```python
from build123d import *

# Parameters (mm, degrees)
SALIENTE_EXTRUIR1_DEPTH = 32
CORTAR_EXTRUIR1_REACH   = 113.66
CROQUIS2_W              = 9.5
CROQUIS2_H              = 13
CORTAR_EXTRUIR2_REACH   = 196.034
REDONDEO2_R             = 16


with BuildPart() as part:
    # Croquis1 → Saliente-Extruir1 (new, symmetric)
    with BuildSketch(Plane.XY):
        with BuildLine():
            Line((-100, 27), (-100, 17))
            Line((-100, 17), (-40, 17))
            Line((-40, 17), (-40, 35))
            ThreePointArc((-40, 35), (-20, 55), (0, 35))
            Line((0, 35), (0, 0))
            Line((0, 0), (80, 0))
            Line((80, 0), (80, 56))
            Line((80, 56), (70, 56))
            Line((70, 56), (70, 10))
            Line((70, 10), (10, 10))
            Line((10, 10), (10, 35))
            ThreePointArc((10, 35), (-20, 65), (-50, 35))
            Line((-50, 35), (-50, 27))
            Line((-50, 27), (-100, 27))
        make_face()
    extrude(amount=SALIENTE_EXTRUIR1_DEPTH, both=True)

    # Croquis2 → Cortar-Extruir1 (cut, up to next)
    with BuildSketch(Plane(origin=(0, 27, 0), x_dir=(1, 0, 0), z_dir=(0, 1, 0)), mode=Mode.PRIVATE) as cortar_extruir1_sk1:
        Polygon((-100, 13.524791386), (-68, 32), (-100, 32), align=None)
    cortar_extruir1_tool1 = extrude(cortar_extruir1_sk1.sketch, amount=-CORTAR_EXTRUIR1_REACH, mode=Mode.PRIVATE) & part.part
    # Croquis2 → Cortar-Extruir1 (cut, up to next)
    with BuildSketch(Plane(origin=(0, 27, 0), x_dir=(1, 0, 0), z_dir=(0, 1, 0)), mode=Mode.PRIVATE) as cortar_extruir1_sk2:
        with Locations((-95.25, 0)):
            Rectangle(CROQUIS2_W, CROQUIS2_H)
    cortar_extruir1_tool2 = extrude(cortar_extruir1_sk2.sketch, amount=-CORTAR_EXTRUIR1_REACH, mode=Mode.PRIVATE) & part.part
    # Croquis2 → Cortar-Extruir1 (cut, up to next)
    with BuildSketch(Plane(origin=(0, 27, 0), x_dir=(1, 0, 0), z_dir=(0, 1, 0)), mode=Mode.PRIVATE) as cortar_extruir1_sk3:
        Polygon((-100, -13.524791386), (-100, -32), (-68, -32), align=None)
    cortar_extruir1_tool3 = extrude(cortar_extruir1_sk3.sketch, amount=-CORTAR_EXTRUIR1_REACH, mode=Mode.PRIVATE) & part.part
    add(cortar_extruir1_tool1.solids().sort_by_distance((-89.333333, 27, -25.841597))[0], mode=Mode.SUBTRACT)
    add(cortar_extruir1_tool2.solids().sort_by_distance((-95.25, 27, 0))[0], mode=Mode.SUBTRACT)
    add(cortar_extruir1_tool3.solids().sort_by_distance((-89.333333, 27, 25.841597))[0], mode=Mode.SUBTRACT)

    # Croquis4 → Cortar-Extruir2 (cut, up to next)
    with BuildSketch(Plane(origin=(80, 0, 0), x_dir=(0, 0, -1), z_dir=(1, 0, 0)), mode=Mode.PRIVATE) as cortar_extruir2_sk1:
        with BuildLine():
            Line((-16, 48.75), (16, 48.75))
            ThreePointArc((16, 48.75), (24.75, 40), (16, 31.25))
            Line((16, 31.25), (-16, 31.25))
            ThreePointArc((-16, 31.25), (-24.75, 40), (-16, 48.75))
        make_face()
    cortar_extruir2_tool1 = extrude(cortar_extruir2_sk1.sketch, amount=-CORTAR_EXTRUIR2_REACH, mode=Mode.PRIVATE) & part.part
    add(cortar_extruir2_tool1.solids().sort_by_distance((80, 40, 0))[0], mode=Mode.SUBTRACT)

    # Redondeo2
    redondeo2_edges = [part.edges().sort_by_distance(p)[0] for p in [
        (75, 56, -32),
        (75, 56, 32),
    ]]
    fillet(redondeo2_edges, radius=REDONDEO2_R)


solid = part.part
```
Input: part model. Units: mm. Frame: model coordinates. A direction names the side the tool comes from. Round coordinates to 2 decimals unless told otherwise and drop trailing zeros. Write each loop counter-clockwise with the first axis right and the second up, starting at its lowest first coordinate (ties: lowest second). Pieces come first, ordered by that corner, then holes. Notation, with made-up numbers: (-5.75, 61.25) -> (45.25, 61.25) arc R13 ccw to (45.25, 71.25) -> close; hole circle Ø1 at (-12, 64.5). An arc over 180 degrees is marked (long way). Answer as CSV lines item,"result".
1. Contact query for flat-ended pins moving along their axis: P1, Ø3, axis at x = -20.5, z = -11.5, coming from the +Y side; P2, Ø17.5, axis at y = 10.5, z = -2.5, coming from the -X side; P3, Ø8, axis at y = 21.5, z = -1, coming from the -X side; P4, Ø4, axis at x = -6.5, z = -6.5, coming from the -Y side. Output: stop coordinate, or through.
Geometry says:
P1,"stops at y = 65"
P2,"stops at x = -100"
P3,"stops at x = -90.5"
P4,"stops at y = 47.64"
2. Ray query, L1, parallel to X at y = 31, z = 8; L2, parallel to X at y = 21.5, z = 1.5; L3, parallel to X at y = 11.5, z = -22. Return the intervals inside material, ascending. Write a range as [from, to].
Geometry says:
L1,"x = [-50, -40], [0, 10], [70, 80]"
L2,"x = [-90.5, -40], [0, 10], [70, 80]"
L3,"x = [0, 10], [70, 80]"
3. Reachability of faces 4 (the flat face through (-90.5, 22, 0)), 5 (the flat face through (-50, 31, 0)), 6 (the cylindrical face through (74.93, 51.189, -27.437)), 7 (the cylindrical face through (75.07, 40.192, -24.748)), 8 (the flat face through (10, 22, 0)) from +Z, -Z, +X, -X, +Y, -Y: full face, straight path, thin tool, end or side. Return the list, or none.
Geometry says:
face 4,"-X, +Y, -Y"
face 5,"+Z, -Z, -X, +Y"
face 6,"-Z, +X, +Y"
face 7,"+X"
face 8,"+Z, -Z, +Y"
4. Mould query, pull axis Z, two halves, no side actions, for faces 1 (the flat face through (-100, 22, 10)), 2 (the flat face through (6, 28, 32)), 3 (the flat face through (75, 48.75, 0)). Classes: +Z half, -Z half, draft (parallel to the pull), parting line (faces both ways), or undercut.
Geometry says:
face 1,"draft"
face 2,"+Z half"
face 3,"undercut"
5. Section C-C (z = -20). Return the cut outline in (x, y).
Geometry says:
outline,"(-88.78, 17) -> (-40, 17) -> (-40, 35) arc R20 cw to (0, 35) -> (0, 0) -> (80, 0) -> (80, 32.22) -> (70, 32.22) -> (70, 10) -> (10, 10) -> (10, 35) arc R30 ccw to (-50, 35) -> (-50, 27) -> (-88.78, 27) -> close; (70, 47.78) -> (80, 47.78) -> (80, 55.49) -> (70, 55.49) -> close"
6. Section A-A (z = -1). Return the cut outline in (x, y).
Geometry says:
outline,"(-90.5, 17) -> (-40, 17) -> (-40, 35) arc R20 cw to (0, 35) -> (0, 0) -> (80, 0) -> (80, 31.25) -> (70, 31.25) -> (70, 10) -> (10, 10) -> (10, 35) arc R30 ccw to (-50, 35) -> (-50, 27) -> (-90.5, 27) -> close; (70, 48.75) -> (80, 48.75) -> (80, 56) -> (70, 56) -> close"
7. Section D-D (x = 59). Return the cut outline in (y, z).
Geometry says:
outline,"(0, -32) -> (10, -32) -> (10, 32) -> (0, 32) -> close"
8. Section B-B (y = 38). Return the cut outline in (x, z).
Geometry says:
outline,"(-49.85, -32) -> (-39.77, -32) -> (-39.77, 32) -> (-49.85, 32) -> close; (-0.23, -32) -> (9.85, -32) -> (9.85, 32) -> (-0.23, 32) -> close; (70, -32) -> (80, -32) -> (80, -24.52) -> (70, -24.52) -> close; (70, 24.52) -> (80, 24.52) -> (80, 32) -> (70, 32) -> close"
